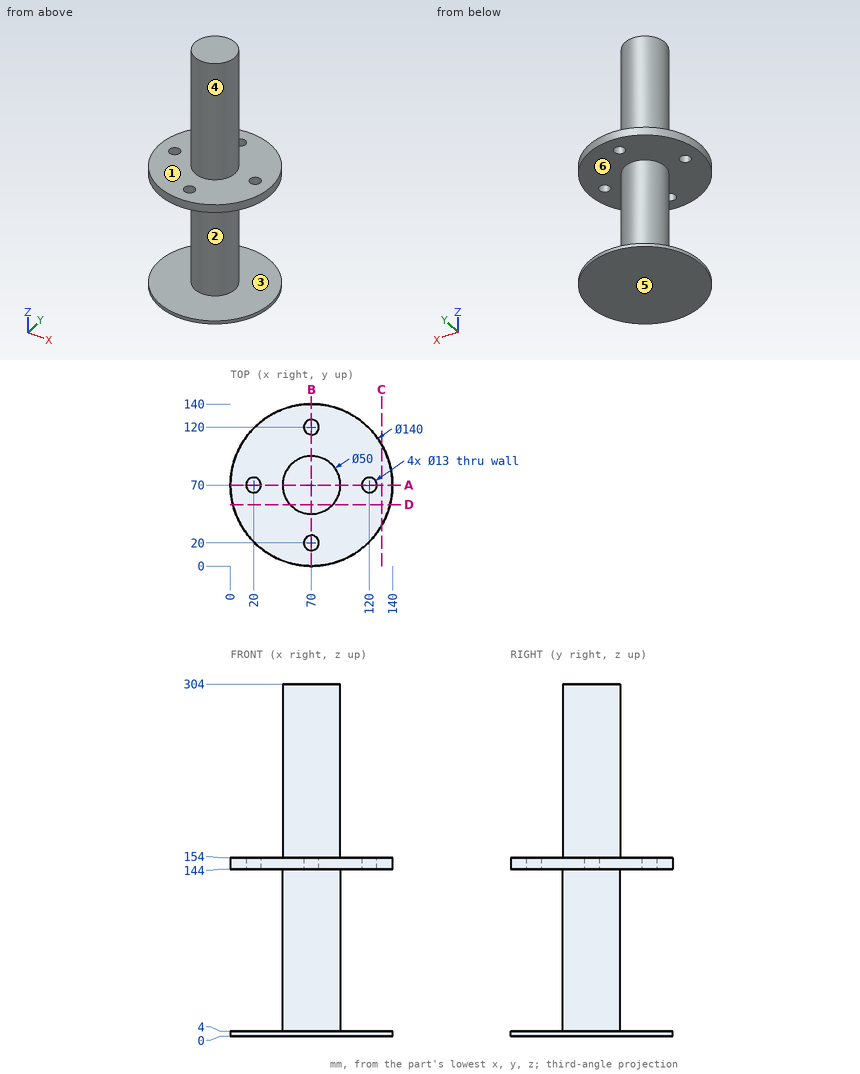
Study the drawing (mm; zero at the part's minimum x, y, z) and answer. A direction names the side the tool comes from. Round coordinates to 2 decimals unless told otherwise and drop trailing zeros. Write each loop counter-clockwise with the first axis right and the second up, starting at its lowest first coordinate (ties: lowest second). Pieces come first, ordered by that corner, then holes.
1) A cutting plane is placed at A-A (y = 70). Give the vertices of the cut face in (x, z).
2) Given pin 1 Ø2 at (x, z) = (65, 88) entering from +Y; pin 2 Ø10.5 at (x, y) = (70, 20) entering from +Z; pin 3 Ø12 at (y, z) = (42.5, 132) entering from +X, each flat-ended and moving along its own axis, determine where each tip first touches the part or whether it passes through.
3) The mould has two halves that part along Z. Classify the marked faces 1, 2, 3 and 4: pulls with the +Z half, pulls with the -Z half, needs draft (parallel to the pull), parting line crosses it, or undercut.
4) A tool of negligible diameter and unlimited length cuts with its end or side. For the marked faces 5 and 6, from which of +Z, -Z, +X, -X, +Y, -Y can it reach the whole face along a straight path? Write none if from no direction.
5) Straight lines are drawn through the part: line 1 (Y direction, x = 70, z = 151); line 2 (Z direction, x = 10.5, y = 106.5); line 3 (Y direction, x = 70, z = 178). For each, find the intervals that lie inside material, in ascending order.
6) A cutting plane is placed at D-D (y = 53). Give the vertices of the cut face in (x, z), plus the area to 3 significant figures.
7) A cutting plane is placed at C-C (x = 130.5). Give the vertices of the cut face in (y, z), plus the area to 3 significant figures.
Completed:
1. outline: (0, 0) - (140, 0) - (140, 4) - (95, 4) - (95, 144) - (113.5, 144) - (113.5, 154) - (95, 154) - (95, 304) - (45, 304) - (45, 154) - (26.5, 154) - (26.5, 144) - (45, 144) - (45, 4) - (0, 4) - close; (0, 144) - (13.5, 144) - (13.5, 154) - (0, 154) - close; (126.5, 144) - (140, 144) - (140, 154) - (126.5, 154) - close
2. pin 1: stops at y = 94.68
2. pin 2: stops at z = 4
2. pin 3: stops at x = 82.76
3. face 1: pulls with the +Z half
3. face 2: undercut
3. face 3: undercut
3. face 4: needs draft
4. face 5: -Z, +X, -X, +Y, -Y
4. face 6: none
5. line 1: y = 0 to 13.5, 26.5 to 113.5, 126.5 to 140
5. line 2: z = 0 to 4, 144 to 154
5. line 3: y = 45 to 95
6. outline: (2.1, 0) - (137.9, 0) - (137.9, 4) - (88.33, 4) - (88.33, 144) - (137.9, 144) - (137.9, 154) - (88.33, 154) - (88.33, 304) - (51.67, 304) - (51.67, 154) - (2.1, 154) - (2.1, 144) - (51.67, 144) - (51.67, 4) - (2.1, 4) - close
6. area: 12,500 mm2
7. outline: (34.79, 0) - (105.21, 0) - (105.21, 4) - (34.79, 4) - close; (34.79, 144) - (105.21, 144) - (105.21, 154) - (34.79, 154) - close
7. area: 986 mm2
